Geometry check sheet. Reference: the model listing, model coordinates, mm. Face numbers are marked on the shaded views. A direction names the side the tool comes from. Coordinates: 2 decimals unless noted, no trailing zeros. Write each loop counter-clockwise with the first axis right and the second up, starting at its lowest first coordinate (ties: lowest second). Pieces come first, ordered by that corner, then holes. Notation, with made-up numbers: (-5, -20.5) -> (10, -20.5) arc R34 cw to (10, 13.5) -> close; hole circle Ø10 at (7, -39). An arc over 180 degrees is marked (long way). Answer in a Markdown table with one row per item. Add a question column.
Q1. Tool access check on the marked faces 1 and 2. Record the directions out of +Z, -Z, +X, -X, +Y, -Y that give a thin tool (end or side, any length) a straight path to the whole face; none if there is none.
Q2. Gauge pin test, flat end, axial feed: P1, Ø2.5, axis at x = 6, y = 1.5, coming from the +Z side. Record the tip position at first contact, or that the pin passes through.
Q3. Section check A-A, the plane x = 9. Record the boundary of the cut face in (y, z).
Q4. Release check for a two-part mould opening along Z. For the marked faces 3, 4 and 5 record: pulls with the +Z half, pulls with the -Z half, needs draft (parallel to the pull), parting line crosses it, or undercut.
Q5. Section check B-B, the plane z = 9. Record the boundary of the cut face in (x, y), and give its area (3 significant figures).
Q6. Section check C-C, the plane y = 3.4. Record the boundary of the cut face in (x, z).
Q7. Thickness scan on line 1 (Y direction, x = 9, z = 0.95); line 2 (X direction, y = 3.1, z = 10.5). Record the ranges inside material, lowest first.
Q8. Section check D-D, the plane y = 0.6. Record the boundary of the cut face in (x, z), and give its area (3 significant figures).
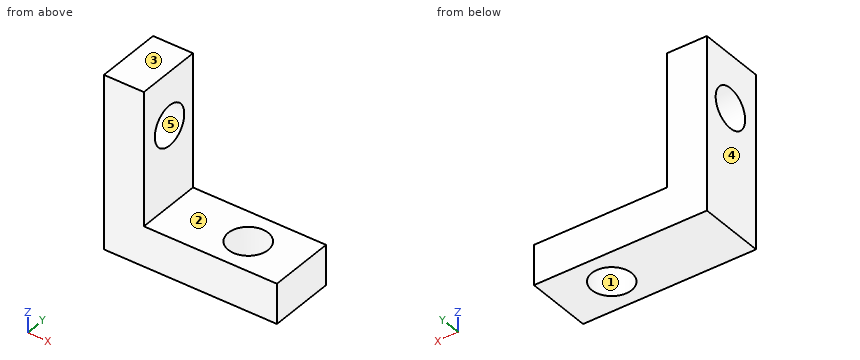
```python
from build123d import *

# Parameters (mm, degrees)
SKETCH_W     = 13
SKETCH_H     = 5
SKETCH_R     = 1.5
PAD_DEPTH    = 3
SKETCH001_W  = 3
SKETCH001_H  = 5
PAD001_DEPTH = 10
SKETCH002_R  = 1.5
POCKET_DEPTH = 13.001


with BuildPart() as part:
    # Sketch → Pad (new body)
    with BuildSketch(Plane.XY):
        with Locations((6.5, 2.5)):
            Rectangle(SKETCH_W, SKETCH_H)
        with Locations((9, 2.5)):
            Circle(SKETCH_R, mode=Mode.SUBTRACT)
    extrude(amount=PAD_DEPTH)

    # Sketch001 → Pad001 (new body)
    with BuildSketch(Plane.XY.offset(3)):
        with Locations((1.5, 2.5)):
            Rectangle(SKETCH001_W, SKETCH001_H)
    extrude(amount=PAD001_DEPTH)

    # Sketch002 → Pocket (cut, through all)
    with BuildSketch(Plane(origin=(0, 0, 0), x_dir=(0, -1, 0), z_dir=(-1, 0, 0))):
        with Locations((-2.610739, 9)):
            Circle(SKETCH002_R)
    extrude(amount=-POCKET_DEPTH, mode=Mode.SUBTRACT)


solid = part.part
```
Calculated:
| question | item | result |
|---|---|---|
| 1 | face 1 | +Z, -Z |
| 1 | face 2 | +Z, +X, +Y, -Y |
| 2 | P1 | stops at z = 3 |
| 3 | outline | (0, 0) -> (1, 0) -> (1, 3) -> (0, 3) -> close; (4, 0) -> (5, 0) -> (5, 3) -> (4, 3) -> close |
| 4 | face 3 | pulls with the +Z half |
| 4 | face 4 | needs draft |
| 4 | face 5 | undercut |
| 5 | outline | (0, 0) -> (3, 0) -> (3, 1.11) -> (0, 1.11) -> close; (0, 4.11) -> (3, 4.11) -> (3, 5) -> (0, 5) -> close |
| 5 | area | 6.00 mm² |
| 6 | outline | (0, 0) -> (7.8, 0) -> (7.8, 3) -> (3, 3) -> (3, 7.72) -> (0, 7.72) -> close; (0, 10.28) -> (3, 10.28) -> (3, 13) -> (0, 13) -> close; (10.2, 0) -> (13, 0) -> (13, 3) -> (10.2, 3) -> close |
| 7 | line 1 | y = 0 to 1, 4 to 5 |
| 7 | line 2 | x = 0 to 3 |
| 8 | outline | (0, 0) -> (13, 0) -> (13, 3) -> (3, 3) -> (3, 13) -> (0, 13) -> close |
| 8 | area | 69.0 mm² |
